Input: part model. Units: mm. Frame: model coordinates. Face numbers are marked on the shaded views. A direction names the side the tool comes from. Coordinates: 2 decimals unless noted, no trailing zeros. Write each loop counter-clockwise with the first axis right and the second up, starting at its lowest first coordinate (ties: lowest second). Pieces come first, ordered by that corner, then holes. Notation, with made-up numbers: (-36, 71.25) -> (-1, 71.25) arc R25 cw to (-1, 89.25) -> close; hole circle Ø5 at (0, 65). An arc over 180 degrees is marked (long way). Use one line per item in the form item = value. Start each with the question number.
(1) Cut plane B-B on y = 14. Return the cut outline in (x, z), plus the area to 3 significant figures.
(2) Pull-direction query (Y, two-part tool) for the marked faces 1, 2 and 3; classes: released by +Y, released by -Y, zero draft, split by the parting line, or undercut.
(3) First-contact query: pin 1 (10 mm diameter, centred on y = -6.5, z = 10, fed in from -X); pin 2 (4 mm diameter, centred on x = -13.5, y = 13, fed in from -Z); pin 3 (3 mm diameter, centred on x = -43.5, z = 20, fed in from -Y); pin 4 (10 mm diameter, centred on y = 13.5, z = 3.5, fed in from +X). Flat tips, straight axial feed; report the tip coordinate or a pass-through.
(4) Ray query, line 1 along Z through (x, y) = (-37, 21.5); line 2 along X through (y, z) = (11.5, 9); line 3 along Y through (x, z) = (-44.5, 22.75). Return the intervals inside material, ascending.
(5) Cut plane A-A on x = 17. Return the cut outline in (y, z).
(6) Set-up query: the marked faces 4, 5 and 6. Return all of +Z, -Z, +X, -X, +Y, -Y with unobstructed straight access to the full face (end or side cutting, diameter ignored); none if empty.
(7) Cut plane C-C on z = 10.5. Return the cut outline in (x, y), plus the area to 3 significant figures.
```python
from build123d import *

# Parameters (mm, degrees)
F0_R     = 44.6905983142
F1_DEPTH = 25
F2_R     = 39.7625811832
F3_DEPTH = 4
F5_DEPTH = 21.001
F6_R     = 0.7154375695
F7_DEPTH = 21.0010001
F8_R     = 39.7662150712
F8_R_2   = 0.7154375695
F9_DEPTH = 14


with BuildPart() as f1:
    # F0 (on Top) → F1 (new body)
    with BuildSketch(Plane.XY):
        with Locations((-15.1616595685, 9.6226148307)):
            Circle(F0_R)
    extrude(amount=F1_DEPTH)

    # F2 (on face) → F3 (cut)
    with BuildSketch(Plane.XY.offset(25)):
        with Locations((-15.1616595685, 9.6226148307)):
            Circle(F2_R)
    extrude(amount=-F3_DEPTH, mode=Mode.SUBTRACT)

    # F4 (on face) → F5 (cut, through all)
    with BuildSketch(Plane.XY.offset(21)):
        with BuildLine():
            add(Edge.make_bspline(
                [(-24.8842015862, -23.9847730845), (-24.751571743, -25.7479147281), (-14.8764070104, -28.1339639947), (2.363229172, -22.8278430113), (-15.4108273297, -17.1809770311), (-25.0192258083, -22.1898012822), (-24.8842015862, -23.9847730845)],
                knots=[0, 0, 0, 0, 0.2396576866, 0.4971175886, 0.7560157511, 1, 1, 1, 1], degree=3))
        make_face()
    extrude(amount=-F5_DEPTH, mode=Mode.SUBTRACT)

    # F6 (on face) → F7 (cut, through all)
    with BuildSketch(Plane.XY.offset(21)):
        with Locations((-15.7932732254, 46.6668978333)):
            Circle(F6_R)
    extrude(amount=-F7_DEPTH, mode=Mode.SUBTRACT)

    # F8 (on face) → F9 (cut)
    with BuildSketch(Plane(origin=(0, 0, 0), x_dir=(1, 0, 0), z_dir=(0, 0, -1))):
        with Locations((-15.1616595685, -9.6226148307)):
            Circle(F8_R)
        with Locations((-15.7932732254, -46.6668978333)):
            Circle(F8_R_2, mode=Mode.SUBTRACT)
        with BuildLine():
            add(Edge.make_bspline(
                [(-24.8842015862, 23.9847730845), (-24.8911452084, 23.8924666388), (-24.888371728, 23.799570827), (-24.8762555423, 23.7072804576), (-24.855790455, 23.6164271336), (-24.8281284381, 23.5275727498), (-24.7943692309, 23.4410534624), (-24.7554721282, 23.3569978115), (-24.6762660636, 23.2076683313), (-24.6373321353, 23.141629018), (-24.5957616183, 23.0771739055), (-24.5518941434, 23.0142517205), (-24.5060146802, 22.9528055987), (-24.4583585563, 22.8927697396), (-24.4091136917, 22.8340678621), (-24.2951335725, 22.7048867825), (-24.2296199391, 22.6351387447), (-24.1621765597, 22.5672221501), (-24.0930442899, 22.5010185723), (-24.0224196237, 22.4364260325), (-23.9504628247, 22.3733507123), (-23.8773019966, 22.3117027052), (-23.6280353269, 22.1092963253), (-23.4470131486, 21.9747437686), (-23.2612685118, 21.8466153281), (-23.0716712534, 21.7242481532), (-22.87886828, 21.6071333648), (-22.6833359387, 21.4948360767), (-22.4853761009, 21.3869997408), (-22.0365992692, 21.1545493655), (-21.7847229546, 21.0322559578), (-21.5300131244, 20.9158571469), (-21.2728395726, 20.8049762518), (-21.0134959265, 20.6993265457), (-20.7522141353, 20.5986781439), (-20.4891682368, 20.502849378), (-19.8972368304, 20.2989876643), (-19.5675375394, 20.1934415753), (-19.2356580968, 20.0947838468), (-18.9018320844, 20.0028445839), (-18.5662614795, 19.9175220072), (-18.2291224443, 19.838762292), (-17.8905679312, 19.7665502585), (-17.2582009761, 19.6444102678), (-16.964736384, 19.5927818802), (-16.6704234935, 19.5460424355), (-16.3753531794, 19.5042292364), (-16.0796172889, 19.4673986596), (-15.7833089045, 19.4356246154), (-15.4865226065, 19.4089970085), (-14.6964867848, 19.3521656766), (-14.2026325717, 19.3311579491), (-13.7082719853, 19.323673936), (-13.2138389543, 19.3290136415), (-12.7197212313, 19.3466491477), (-12.2262608224, 19.3762031344), (-11.7337550637, 19.4174569261), (-10.813518073, 19.5166010712), (-10.3855908509, 19.5717051597), (-9.9588285875, 19.6356829877), (-9.5334400248, 19.7086182547), (-9.109697804, 19.7907216797), (-8.6879395492, 19.8823360076), (-8.2685809043, 19.9840006907), (-7.6692511074, 20.1461394501), (-7.4869229926, 20.197739325), (-7.305219405, 20.2515355676), (-7.1241991626, 20.3076214003), (-6.9439349033, 20.3661052757), (-6.7645147562, 20.4271160266), (-6.5860453938, 20.4908121068), (-6.254696052, 20.6151838585), (-6.1015679798, 20.6751409609), (-5.9493429971, 20.7374007127), (-5.7981254711, 20.8021210424), (-5.6480527105, 20.8694825334), (-5.4993000619, 20.9396997859), (-5.352091776, 21.0130449311), (-5.049328083, 21.1730724882), (-4.8944301935, 21.2601773381), (-4.7420379458, 21.351804078), (-4.5925696804, 21.4486212058), (-4.4467809482, 21.5512951436), (-4.3059967032, 21.6607552403), (-4.171918878, 21.7779694123), (-3.9820103602, 21.9721649834), (-3.91933381, 22.0417830638), (-3.859860511, 22.1143746793), (-3.8042449113, 22.190231403), (-3.7534261664, 22.2695356098), (-3.7086220132, 22.352355558), (-3.6712765509, 22.4386130462), (-3.6325609686, 22.5604796694), (-3.6235475081, 22.592989586), (-3.6158562116, 22.625508139), (-3.6094987647, 22.6580310997), (-3.6044868395, 22.690554248), (-3.6008320948, 22.7230733726), (-3.5985461757, 22.7555842705), (-3.5967352526, 22.8205812138), (-3.5972089492, 22.8530673208), (-3.5990503765, 22.8855383141), (-3.6022481072, 22.9179914392), (-3.6067907142, 22.9504239415), (-3.6126667703, 22.9828330664), (-3.619864848, 23.0152160594), (-3.6428351371, 23.102560259), (-3.6608525682, 23.1565906194), (-3.6821125308, 23.2094824212), (-3.7062697452, 23.2611273323), (-3.7329838201, 23.3114710781), (-3.7619452523, 23.3605016698), (-3.7928905413, 23.408242296), (-3.8646571625, 23.5102606567), (-3.9062117551, 23.5639870404), (-3.949907681, 23.6160285277), (-3.995440574, 23.6664779113), (-4.0425578215, 23.7154257906), (-4.0910543201, 23.7629642703), (-4.140770382, 23.8091888469), (-4.2558032479, 23.9110669108), (-4.3217455541, 23.9659664387), (-4.3891611489, 24.0190785563), (-4.4578435397, 24.070548321), (-4.5276265311, 24.120498277), (-4.5983770003, 24.1690378707), (-4.6699912206, 24.2162683608), (-4.8598647658, 24.3369393694), (-4.979368245, 24.4083687716), (-5.1005551521, 24.4769559223), (-5.2231590563, 24.5429853098), (-5.3469747233, 24.606681357), (-5.4718435874, 24.6682345898), (-5.5976470884, 24.7278140349), (-5.8731020203, 24.8534095069), (-6.0230481389, 24.9187177349), (-6.1739919373, 24.9817193826), (-6.3258095179, 25.0425942529), (-6.4784007471, 25.1014892666), (-6.6316847131, 25.1585296043), (-6.7855972746, 25.2138248228), (-7.2450409477, 25.3733585476), (-7.5522097036, 25.4728034138), (-7.8612095316, 25.5665353033), (-8.1717534402, 25.6550457013), (-8.4836197787, 25.7387057177), (-8.7966397248, 25.8178093289), (-9.1106941619, 25.8925843063), (-9.7751521214, 26.0415643167), (-10.1257377207, 26.1148049283), (-10.4773290394, 26.1831793836), (-10.8298122723, 26.2468536908), (-11.1830903824, 26.3059373134), (-11.5370805939, 26.3604964973), (-11.8917133021, 26.410560103), (-12.4141126322, 26.4775592691), (-12.5814208468, 26.4980023592), (-12.7488502783, 26.517446117), (-12.916394228, 26.535887619), (-13.0840460673, 26.5533221125), (-13.2517992377, 26.569743015), (-13.4196472511, 26.5851419147), (-13.755440419, 26.6138684058), (-13.9233852036, 26.6271967172), (-14.0914117258, 26.6394844457), (-14.2595133059, 26.6507169279), (-14.4276829989, 26.6608821201), (-14.5959136343, 26.6699648285), (-14.7641978026, 26.6779426226), (-15.4668094045, 26.7065616899), (-16.0014815913, 26.717052595), (-16.5363439033, 26.7163761275), (-17.0711513874, 26.7044794526), (-17.6056107666, 26.6811276526), (-18.1393801372, 26.6459021949), (-18.6720648144, 26.5981210663), (-19.4381711152, 26.509353217), (-19.6728205121, 26.4794361441), (-19.9071102034, 26.4467241944), (-20.1409861033, 26.4110930398), (-20.374379842, 26.3723961579), (-20.607207594, 26.3304577799), (-20.8393678801, 26.2850600584), (-21.2714530924, 26.1932991389), (-21.4715479801, 26.1478661938), (-21.6709615908, 26.0994400371), (-21.8695961986, 26.0478050892), (-22.067313537, 25.9927020038), (-22.2639323316, 25.9338188721), (-22.4592205165, 25.8707637255), (-22.8526079279, 25.7330984996), (-23.0501942229, 25.658329585), (-23.2457129866, 25.5779976939), (-23.4388079377, 25.4912718478), (-23.6287503173, 25.3972628999), (-23.8142215655, 25.2946773515), (-23.993488719, 25.1821020816), (-24.2354137555, 25.0033783334), (-24.305527566, 24.9480349583), (-24.3736940108, 24.890201273), (-24.4395833556, 24.8296527893), (-24.5027360604, 24.7661764981), (-24.5625646396, 24.6995727976), (-24.6183569307, 24.6296586324), (-24.7132853809, 24.4928564182), (-24.7536853284, 24.4268044353), (-24.7898357294, 24.358145571), (-24.8210372692, 24.2870046025), (-24.8465837183, 24.2136183714), (-24.8658479214, 24.138366296), (-24.8784062595, 24.0618144324), (-24.8842015862, 23.9847730845)],
                knots=[0, 0, 0, 0, 0, 0, 0, 0, 0, 0.0154781502, 0.0154781502, 0.0154781502, 0.0154781502, 0.0154781502, 0.0154781502, 0.0154781502, 0.0283061693, 0.0283061693, 0.0283061693, 0.0283061693, 0.0283061693, 0.0283061693, 0.0283061693, 0.0443208042, 0.0443208042, 0.0443208042, 0.0443208042, 0.0443208042, 0.0443208042, 0.0443208042, 0.0820556467, 0.0820556467, 0.0820556467, 0.0820556467, 0.0820556467, 0.0820556467, 0.0820556467, 0.1289005454, 0.1289005454, 0.1289005454, 0.1289005454, 0.1289005454, 0.1289005454, 0.1289005454, 0.1868172217, 0.1868172217, 0.1868172217, 0.1868172217, 0.1868172217, 0.1868172217, 0.1868172217, 0.2366703877, 0.2366703877, 0.2366703877, 0.2366703877, 0.2366703877, 0.2366703877, 0.2366703877, 0.3193543861, 0.3193543861, 0.3193543861, 0.3193543861, 0.3193543861, 0.3193543861, 0.3193543861, 0.3915439512, 0.3915439512, 0.3915439512, 0.3915439512, 0.3915439512, 0.3915439512, 0.3915439512, 0.4232521415, 0.4232521415, 0.4232521415, 0.4232521415, 0.4232521415, 0.4232521415, 0.4232521415, 0.4507724944, 0.4507724944, 0.4507724944, 0.4507724944, 0.4507724944, 0.4507724944, 0.4507724944, 0.4805674531, 0.4805674531, 0.4805674531, 0.4805674531, 0.4805674531, 0.4805674531, 0.4805674531, 0.496271474, 0.496271474, 0.496271474, 0.496271474, 0.496271474, 0.496271474, 0.496271474, 0.5019818537, 0.5019818537, 0.5019818537, 0.5019818537, 0.5019818537, 0.5019818537, 0.5019818537, 0.5076922315, 0.5076922315, 0.5076922315, 0.5076922315, 0.5076922315, 0.5076922315, 0.5076922315, 0.5173977756, 0.5173977756, 0.5173977756, 0.5173977756, 0.5173977756, 0.5173977756, 0.5173977756, 0.5289826305, 0.5289826305, 0.5289826305, 0.5289826305, 0.5289826305, 0.5289826305, 0.5289826305, 0.5436197749, 0.5436197749, 0.5436197749, 0.5436197749, 0.5436197749, 0.5436197749, 0.5436197749, 0.5673675977, 0.5673675977, 0.5673675977, 0.5673675977, 0.5673675977, 0.5673675977, 0.5673675977, 0.5952652382, 0.5952652382, 0.5952652382, 0.5952652382, 0.5952652382, 0.5952652382, 0.5952652382, 0.6503316105, 0.6503316105, 0.6503316105, 0.6503316105, 0.6503316105, 0.6503316105, 0.6503316105, 0.7114170742, 0.7114170742, 0.7114170742, 0.7114170742, 0.7114170742, 0.7114170742, 0.7114170742, 0.7401663215, 0.7401663215, 0.7401663215, 0.7401663215, 0.7401663215, 0.7401663215, 0.7401663215, 0.7689019232, 0.7689019232, 0.7689019232, 0.7689019232, 0.7689019232, 0.7689019232, 0.7689019232, 0.8601091042, 0.8601091042, 0.8601091042, 0.8601091042, 0.8601091042, 0.8601091042, 0.8601091042, 0.9004581455, 0.9004581455, 0.9004581455, 0.9004581455, 0.9004581455, 0.9004581455, 0.9004581455, 0.9354610916, 0.9354610916, 0.9354610916, 0.9354610916, 0.9354610916, 0.9354610916, 0.9354610916, 0.9715626919, 0.9715626919, 0.9715626919, 0.9715626919, 0.9715626919, 0.9715626919, 0.9715626919, 0.9868177281, 0.9868177281, 0.9868177281, 0.9868177281, 0.9868177281, 0.9868177281, 0.9868177281, 1, 1, 1, 1, 1, 1, 1, 1, 1], degree=8))
        make_face(mode=Mode.SUBTRACT)
    extrude(amount=-F9_DEPTH, mode=Mode.SUBTRACT)


solid = f1.part
```
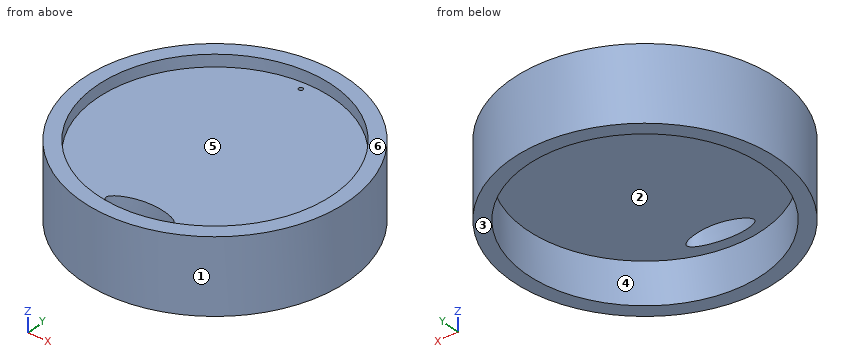
Values:
q1.outline = (-59.64, 0) -> (-54.69, 0) -> (-54.69, 14) -> (24.36, 14) -> (24.36, 0) -> (29.31, 0) -> (29.31, 25) -> (24.36, 25) -> (24.36, 21) -> (-54.68, 21) -> (-54.68, 25) -> (-59.64, 25) -> close
q1.area = 801 mm2
q2.face_1 = split by the parting line
q2.face_2 = undercut
q2.face_3 = zero draft
q3.pin_1 = -58.45
q3.pin_2 = 14
q3.pin_3 = -26.11
q3.pin_4 = 29.53
q4.line_1 = 14 to 21
q4.line_2 = -59.81 to -54.88, 24.56 to 29.49
q4.line_3 = -24.09 to -17.22, 36.46 to 43.33
q5.outline = (-21.41, 0) -> (-13.76, 0) -> (-13.76, 14) -> (33.01, 14) -> (33.01, 0) -> (40.65, 0) -> (40.65, 25) -> (33, 25) -> (33, 21) -> (-13.76, 21) -> (-13.76, 25) -> (-21.41, 25) -> close
q6.face_4 = -Z
q6.face_5 = +Z
q6.face_6 = +Z, +X, -X, +Y, -Y
q7.outline = circle Ø89.38 at (-15.16, 9.62); hole circle Ø79.53 at (-15.16, 9.62)
q7.area = 1,310 mm2
